```python
from build123d import *

# Parameters (mm, degrees)
CROQUIS1_R              = 2.228578899
SALIENTE_EXTRUIR1_DEPTH = 1
SALIENTE_EXTRUIR2_DEPTH = 1
CROQUIS4_R              = 2
CORTAR_EXTRUIR1_DEPTH   = 7


with BuildPart() as part:
    # Croquis1 → Saliente-Extruir1 (new body)
    with BuildSketch(Plane(origin=(0, 0, 0), x_dir=(1, 0, 0), z_dir=(0, 1, 0))):
        with BuildLine():
            Line((-41.112087634, 5.337620698), (-41.112087634, 1.105825587))
            ThreePointArc((-41.112087634, 1.105825587), (-41.131019498, 1.025469781), (-41.183832696, 0.962017144))
            ThreePointArc((-41.183832696, 0.962017144), (-41.639608895, 0.827195653), (-42.072087634, 1.024352746))
            ThreePointArc((-42.072087634, 1.024352746), (-42.672087634, 0.424352746), (-42.072087634, -0.175647254))
            ThreePointArc((-42.072087634, -0.175647254), (-41.6683089, 0.018882448), (-41.231302611, -0.080639282))
            ThreePointArc((-41.231302611, -0.080639282), (-41.143877149, -0.173022759), (-41.112087634, -0.296178535))
            Line((-41.112087634, -0.296178535), (-41.112087634, -5.84119357))
            ThreePointArc((-41.112087634, -5.84119357), (-41.186615392, -6.021119495), (-41.366541317, -6.095647254))
            Line((-41.366541317, -6.095647254), (-61.33763395, -6.095647254))
            ThreePointArc((-61.33763395, -6.095647254), (-61.517559875, -6.021119495), (-61.592087634, -5.84119357))
            Line((-61.592087634, -5.84119357), (-61.592087634, -0.296178535))
            ThreePointArc((-61.592087634, -0.296178535), (-61.560298119, -0.173022759), (-61.472872656, -0.080639282))
            ThreePointArc((-61.472872656, -0.080639282), (-61.035866368, 0.018882448), (-60.632087634, -0.175647254))
            ThreePointArc((-60.632087634, -0.175647254), (-60.032087634, 0.424352746), (-60.632087634, 1.024352746))
            ThreePointArc((-60.632087634, 1.024352746), (-61.064566372, 0.827195653), (-61.520342572, 0.962017144))
            ThreePointArc((-61.520342572, 0.962017144), (-61.57315577, 1.025469781), (-61.592087634, 1.105825587))
            Line((-61.592087634, 1.105825587), (-61.592087634, 5.337620698))
            ThreePointArc((-61.592087634, 5.337620698), (-61.552355908, 5.457262162), (-61.448946833, 5.529368009))
            ThreePointArc((-61.448946833, 5.529368009), (-51.352087634, 6.994851774), (-41.255228435, 5.529368009))
            ThreePointArc((-41.255228435, 5.529368009), (-41.151819359, 5.457262162), (-41.112087634, 5.337620698))
        make_face()
        with Locations((-51.352087634, 3.221723142)):
            Circle(CROQUIS1_R, mode=Mode.SUBTRACT)
    extrude(amount=SALIENTE_EXTRUIR1_DEPTH)

    # Croquis3 → Saliente-Extruir2 (add)
    with BuildSketch(Plane.XY.offset(6.095647254)):
        with BuildLine():
            Line((-61.592087634, 0), (-61.592087634, 13))
            ThreePointArc((-61.592087634, 13), (-51.352087634, 17.241546879), (-41.112087634, 13))
            Line((-41.112087634, 13), (-41.112087634, 0))
            Line((-41.112087634, 0), (-61.592087634, 0))
        make_face()
    extrude(amount=-SALIENTE_EXTRUIR2_DEPTH)

    # Croquis4 → Cortar-Extruir1 (cut)
    with BuildSketch(Plane(origin=(0, 0, 5.095647254), x_dir=(-1, 0, 0), z_dir=(0, 0, -1))):
        with Locations((51.352087634, 13)):
            Circle(CROQUIS4_R)
    extrude(amount=-CORTAR_EXTRUIR1_DEPTH, mode=Mode.SUBTRACT)


solid = part.part
```
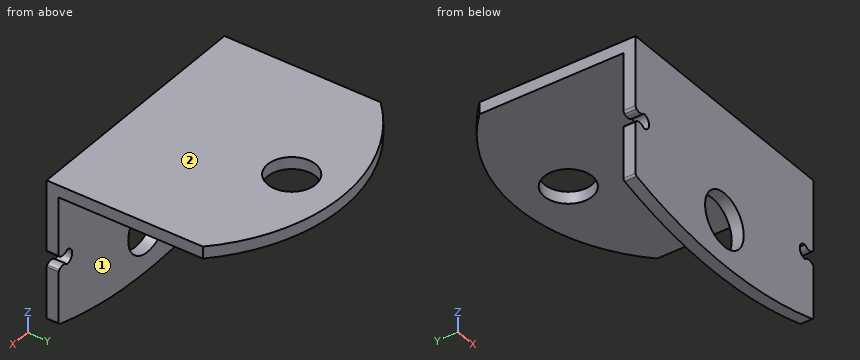
Work out the finished part from the listing and answer in its coordinate system (mm). Face numbers are marked on the shaded views. A direction names the side the tool comes from. Give positions to 0.01 mm unless a question says otherwise; leave off trailing zeros. Order: outer loops, then holes, each group sorted by start corner. A loop starts at its lowest first (then second) coordinate and runs counter-clockwise, first axis right, second up. Notation, with made-up numbers: M 17,74 L 43,74 A21 cw 43,110 Z; hole C 16.5,51.5 d6. An arc over 180 degrees is marked long. Return JSON: item names as keys, results as strings.
1) Section C-C, the plane x = -50 is taken. Write down the section's boundary in (y, z).
Resolved:
{"outline": "M 0,-6.97 L 1,-6.97 L 1,-4.99 L 0,-4.99 Z; M 0,-1.45 L 1,-1.45 L 1,5.1 L 11.53,5.1 L 11.53,6.1 L 0,6.1 Z; M 14.47,5.1 L 17.18,5.1 L 17.18,6.1 L 14.47,6.1 Z"}
2) Section A-A, the plane z = -4.25 is taken. Write down the section's boundary in (x, y).
Resolved:
{"outline": "M -61.59,0 L -53.33,0 L -53.33,1 L -61.59,1 Z; M -49.37,0 L -41.11,0 L -41.11,1 L -49.37,1 Z"}
3) Each of these flat-tipped pins is pushed along its axis until it touches: pin 1 (1 mm diameter, centred on x = -47.5, y = 6.5, fed in from -Z); pin 2 (2 mm diameter, centred on x = -52.5, z = -5.5, fed in from -Y); pin 3 (6 mm diameter, centred on y = 5, z = -0.5, fed in from -X). Where does it stop, or does it pass through?
Resolved:
{"pin 1": "z = 5.1", "pin 2": "y = 0", "pin 3": "through"}
4) Section B-B, the plane y = 12 is taken. Write down the section's boundary in (x, z).
Resolved:
{"outline": "M -61.59,5.1 L -53.08,5.1 L -53.08,6.1 L -61.59,6.1 Z; M -49.62,5.1 L -41.11,5.1 L -41.11,6.1 L -49.62,6.1 Z"}
5) Straight lines are drawn through the part: line 1 along Y through (x, z) = (-48.75, -5); line 2 along Z through (x, y) = (-59.75, 5). For each, find the intervals that lie inside material, in ascending order. Write a range as [from, to].
Resolved:
{"line 1": "[0, 1]", "line 2": "[5.1, 6.1]"}
6) Section D-D, the plane y = 6.25 is taken. Write down the section's boundary in (x, z), plus the area to 3 significant figures.
Resolved:
{"outline": "M -61.59,5.1 L -41.11,5.1 L -41.11,6.1 L -61.59,6.1 Z", "area": "20.5 mm^2"}
7) A tool of negligible diameter and unlimited length cuts with its end or side. For the marked faces 1 and 2, from which of +Z, -Z, +X, -X, +Y, -Y can it reach the whole face along a straight path? Write none if from no direction.
Resolved:
{"face 1": "-Z, +X, -X, +Y", "face 2": "+Z, +X, -X, +Y, -Y"}
